from build123d import *

# Parameters (mm, degrees)
FILLET1_R = 5.08
FILLET2_R = 2.54


with BuildPart() as part:
    # Sketch1 → Revolve1 (revolve)
    with BuildSketch(Plane(origin=(0, 0, 0), x_dir=(0, 0, -1), z_dir=(1, 0, 0)), mode=Mode.PRIVATE) as revolve1_sk:
        with BuildLine():
            Line((-18.244148936, 11.1), (0, 11.557))
            ThreePointArc((0, 11.557), (4.287180767, 13.00922662), (6.994234772, 16.637))
            Line((6.994234772, 16.637), (23.177729058, 16.637))
            Line((23.177729058, 16.637), (23.177729058, 11.557))
            Line((23.177729058, 11.557), (7.937729058, 11.557))
            Line((7.937729058, 11.557), (7.937729058, 7.5))
            Line((7.937729058, 7.5), (-18.244148936, 7.7))
            Line((-18.244148936, 7.7), (-18.244148936, 11.1))
        make_face()
    revolve(revolve1_sk.sketch.rotate(Axis((0, 0, 18.244148936), (0, 0, -1)), 180), axis=Axis((0, 0, 18.244148936), (0, 0, -1)))

    # Fillet1
    # the kernel refuses this fillet: 5.08 mm, written as the material it takes off along each edge
    with BuildSketch(Plane(origin=(0, 0, -7.937729058), x_dir=(0, -1, 0), z_dir=(1, 0, 0))) as fillet1_piece_1:
        with BuildLine():
            CenterArc((12.618097701, -4.967944411), FILLET1_R, 102.056579011, 78.38108757)
            Line((7.53824591, -5.006748745), (7.436648874, -5.007524832))
            Line((7.436648874, -5.007524832), (7.398402964, -0.000776087))
            Line((7.398402964, -0.000776087), (7.5, 0.1016))
            ThreePointArc((7.5, 0.1016), (9.5285, 0.1016), (11.535778046, 0.099358888))
            Line((11.535778046, 0.099358888), (11.557, 0))
        make_face()
    revolve(axis=Axis((0, 0, -7.937729058), (0, 0, -1)), mode=Mode.SUBTRACT)

    # Fillet2
    fillet2_edges = [part.edges().sort_by_distance(p)[0] for p in [
        (0, 16.637, -23.177729058),
        (0, 16.637, -6.994234772),
    ]]
    fillet(fillet2_edges, radius=FILLET2_R)


solid = part.part
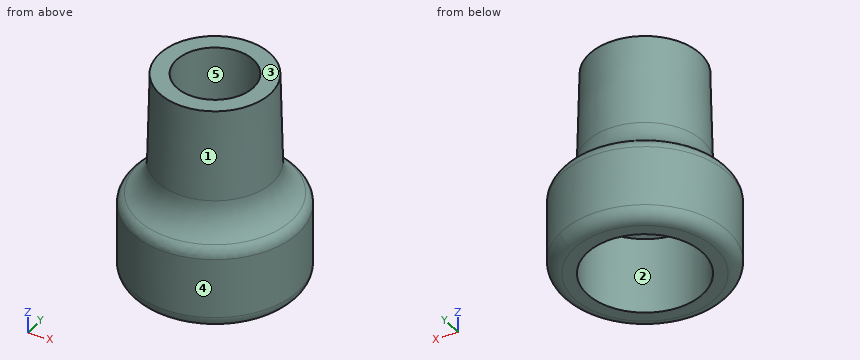
CAD build for the part. Positions are in the model's coordinates, mm. Face numbers are marked on the shaded views. A direction names the side the tool comes from. Give positions to 0.01 mm unless a question says otherwise; leave off trailing zeros. Write each loop counter-clockwise with the first axis right and the second up, starting at its lowest first coordinate (ties: lowest second). Pieces come first, ordered by that corner, then holes. Notation, with made-up numbers: (65.25, 49) - (115.25, 49) arc R9 ccw to (115.25, 60) - close; hole circle Ø6 at (-13.75, -3.75). An arc over 180 degrees is marked (long way). Put each result on its own line as item: value.
(1) Tool access for the marked faces 1 and 2: list every direction of +Z, -Z, +X, -X, +Y, -Y with a clear straight run to the whole face (end or side of a thin tool).
Working result:
face 1: +Z
face 2: -Z
(2) Saw through at B-B (z = 12). List the corners of the cut face in (x, y), then the cut area to 3 significant figures.
Working result:
outline: circle Ø22.51 at (0, 0); hole circle Ø15.3 at (0, 0)
area: 214 mm^2
(3) Drop flat-ended pins along their axis: pin 1 Ø3 at (x, z) = (1, -5) entering from +Y; pin 2 Ø4 at (y, z) = (6.5, -17) entering from -X; pin 3 Ø5 at (y, z) = (-5.5, 5.5) entering from +X; pin 4 Ø4 at (x, y) = (-5, 2) entering from +Z. Give the stop position or say it passes through.
Working result:
pin 1: y = 15.48
pin 2: x = -16.02
pin 3: x = 11.02
pin 4: through
(4) Wall check: L1, parallel to X at y = 0, z = -15; L2, parallel to X at y = 0.5, z = -11; L3, parallel to Y at x = 6, z = -18. Give the ranges that are in metal, low to high.
Working result:
L1: -16.64 to -11.56, 11.56 to 16.64
L2: -16.63 to -11.55, 11.55 to 16.63
L3: -15.52 to -9.88, 9.88 to 15.52
(5) Saw through at A-A (z = -18). List the corners of the cut face in (x, y), then the cut area to 3 significant figures.
Working result:
outline: circle Ø33.27 at (0, 0); hole circle Ø23.11 at (0, 0)
area: 450 mm^2
(6) Pull direction Y, two halves, no side cores. Call the marked faces 3, 4 and 5: released by +Y, released by -Y, zero draft, split by the parting line, or undercut.
Working result:
face 3: zero draft
face 4: split by the parting line
face 5: undercut
